from build123d import *

# Parameters (mm, degrees)
SKETCH3_R             = 21.5
BOSS_EXTRUDE3_DEPTH   = 1
F_5_0MM_DOWEL_HOLE1_D = 5


with BuildPart() as part:
    # Sketch3 → Boss-Extrude3 (new body)
    with BuildSketch(Plane(origin=(0, 0, 0), x_dir=(1, 0, 0), z_dir=(0, 1, 0))):
        with BuildLine():
            Line((-147.74649939, -18.972612677), (148.057489765, -18.972612677))
            ThreePointArc((148.057489765, -18.972612677), (0.155495187, 106.027387323), (-147.74649939, -18.972612677))
        make_face()
        with Locations(Location((-96.926544138, 26.561617598, 0), (0, 0, 270))):
            Circle(SKETCH3_R, mode=Mode.SUBTRACT)
        with Locations(Location((97.237534512, 26.561617598, 0), (0, 0, 270))):
            Circle(SKETCH3_R, mode=Mode.SUBTRACT)
        with Locations(Location((-36.926544138, 70.154169278, 0), (0, 0, 270))):
            Circle(SKETCH3_R, mode=Mode.SUBTRACT)
        with Locations(Location((37.237534512, 70.154169278, 0), (0, 0, 270))):
            Circle(SKETCH3_R, mode=Mode.SUBTRACT)
    extrude(amount=BOSS_EXTRUDE3_DEPTH)

    # Ø5.0mm Dowel Hole1 (through all)
    with Locations(Plane(origin=(0, 0, 0), x_dir=(-1, 0, 0), z_dir=(0, -1, 0))):
        with Locations((-97.237534512, 56.561617598), (-67.237534512, 26.561617598), (-67.237534512, 70.154169278), (-7.237534512, 70.154169278), (6.926544138, 70.154169278), (66.926544138, 70.154169278), (96.926544138, 56.561617598), (66.926544138, 26.561617598)):
            Hole(F_5_0MM_DOWEL_HOLE1_D / 2)


solid = part.part
Verification items for the finished model (mm, model axes). Give positions to 0.01 mm unless a question says otherwise; leave off trailing zeros. Loops run counter-clockwise (first coordinate to the right, second up) from the corner with the lowest first, then second, coordinate; pieces in that order, holes last.
1. Cross-section at D-D on x = 43. Record the cut outline in (y, z), and give its area (3 significant figures).
Derived:
outline: (0, -99.78) - (1, -99.78) - (1, -90.87) - (0, -90.87) - close; (0, -49.44) - (1, -49.44) - (1, 18.97) - (0, 18.97) - close
area: 77.3 mm2
2. Cross-section at C-C on y = 0.4. Count the separate pieces of the cut face and the enclosed holes in it, and give its area (3 significant figures).
Derived:
separate pieces: 1
enclosed holes: 12
area: 21,900 mm2
3. Cross-section at B-B on x = -105.5. Record the cut outline in (y, z).
Derived:
outline: (0, -62.5) - (1, -62.5) - (1, -46.28) - (0, -46.28) - close; (0, -6.84) - (1, -6.84) - (1, 18.97) - (0, 18.97) - close
4. Material ranges on probe 1 along X at (y, z) = (0.5, -13.5); probe 2 along X at (y, z) = (0.45, -7.5); probe 3 along Z at (x, y) = (68.5, 0.15), recorded low to high.
Derived:
probe 1: x = -138.4 to -114, -79.85 to 80.16, 114.32 to 138.71
probe 2: x = -140.74 to -106.87, -86.98 to 87.29, 107.18 to 141.05
probe 3: z = -89.55 to -72.31, -68 to -28.72, -24.4 to 18.97
5. Go/stop test with a flat-tipped pin: P1, Ø3, axis at x = 67.24, z = -70.15, coming from the +Y side. Record where the tip stops, or that it passes through.
Derived:
P1: passes through
6. Cross-section at A-A on z = -9.5. Record the cut outline in (x, y).
Derived:
outline: (-139.99, 0) - (-110.01, 0) - (-110.01, 1) - (-139.99, 1) - close; (-83.84, 0) - (84.16, 0) - (84.16, 1) - (-83.84, 1) - close; (110.32, 0) - (140.3, 0) - (140.3, 1) - (110.32, 1) - close
7. Release check for a two-part mould opening along X. For faces 1 (the cylindrical face through (95.395, 0.507, -58.251)), 2 (the cylindrical face through (3.1, 0.5, -106)), 3 (the flat face through (-2, 1, -31)) record: +X half, -X half, draft (parallel to the pull), parting line (faces both ways), or undercut.
Derived:
face 1: undercut
face 2: parting line
face 3: draft
